Geometry check sheet. Reference: the model listing, model coordinates, mm. Round coordinates to 2 decimals unless told otherwise and drop trailing zeros. Write each loop counter-clockwise with the first axis right and the second up, starting at its lowest first coordinate (ties: lowest second). Pieces come first, ordered by that corner, then holes.
Item 1: Cross-section at B-B (z = 83.5). Enter the section's corners in (x, y), then the cut area to 3 significant figures.
Item 2: Depth check by flat-ended pin: P1, Ø18, axis at x = 0, y = 0, coming from the -Z side; P2, Ø1, axis at x = -10, z = 80.5, coming from the -Y side; P3, Ø12, axis at y = -12.5, z = 71, coming from the +X side; P4, Ø5, axis at x = 0, y = 0, coming from the +Z side. Enter the tip coordinate at first touch or a pass-through.
Item 3: Cross-section at A-A (x = 0). State how many separate pieces and enclosed holes the cut face has, then the cut area to 3 significant figures.
Item 4: Scan lines: probe 1 along X at (y, z) = (-0.5, 69); probe 2 along Y at (x, z) = (0, 149.75); probe 3 along Y at (x, z) = (0, 76.5). Record each from-to range of solid material in increasing order.
from build123d import *

# Parameters (mm, degrees)
F0_R      = 25.4
F1_DEPTH  = 152.5
F2_T      = -2.5
F3_R      = 6.5
F4_DEPTH  = 150
F5_T      = -2.5
F6_R      = 13.75
F7_DEPTH  = 12
F8_R      = 11.25
F11_DEPTH = 10
F12_R     = 25.4
F13_DEPTH = 2.5
F14_R     = 13.75
F15_DEPTH = 12.5
F16_R     = 11.25
F17_DEPTH = 10
F18_R     = 4
F19_DEPTH = 142.501
F20_R     = 3
F21_DEPTH = 25


# Not quite as in the source:
# - a fillet or chamfer that OpenCascade refuses, or shapes differently, is made with other operations: its cross-section is extruded or revolved along the edge and cut away or added


with BuildPart() as f1:
    # F0 (on Top) → F1 (new body)
    with BuildSketch(Plane.XY):
        Circle(F0_R)
    extrude(amount=F1_DEPTH)

    # F2
    f2_openings = [f1.faces().sort_by_distance(p)[0] for p in [
        (0, 0, 152.5),
    ]]
    offset(amount=F2_T, openings=f2_openings)

    # F3 (on face) → F4 (join)
    with BuildSketch(Plane.XY.offset(2.5)):
        Circle(F3_R)
    extrude(amount=F4_DEPTH)

    # F5: a shell. OpenCascade refuses it in one call, so the cavity is built on its own and cut out:
    # the body offset inwards by the wall thickness, plus a prism from it out through each open face.
    f5_core = offset(f1.part, amount=F5_T, kind=Kind.INTERSECTION, mode=Mode.PRIVATE)
    f5_exits = [f5_core.faces().sort_by_distance(p)[0] for p in [
        (0, 0, 150),
    ]]
    add(f5_core, mode=Mode.SUBTRACT)
    extrude(f5_exits, amount=-F5_T, mode=Mode.SUBTRACT)

    # F6 (on face) → F7 (join)
    with BuildSketch(Plane(origin=(0, 0, 0), x_dir=(1, 0, 0), z_dir=(0, 0, -1))):
        Circle(F6_R)
    extrude(amount=-F7_DEPTH)

    # F9: fillet of radius 10 on 1 edges, made by hand

    # F9_s1 → F9_t2 (revolve)
    with BuildSketch(Plane.XZ):
        with BuildLine():
            ThreePointArc((22.9, 12.4638095124), (20.2654599313, 5.6999348832), (13.75, 2.5))
            Line((13.75, 2.5), (22.9, 2.5))
            Line((22.9, 2.5), (22.9, 12.4638095124))
        make_face()
    revolve(axis=Axis((0, 0, 2.5), (0, 0, -1)))

    # F10: fillet of radius 8 on 1 edges, made by hand

    # F10_s1 → F10_t2 (revolve)
    with BuildSketch(Plane.XZ):
        with BuildLine():
            ThreePointArc((13.75, 12), (8.5839202169, 14.5796013539), (6.5, 19.964766161))
            Line((6.5, 19.964766161), (6.5, 12))
            Line((6.5, 12), (13.75, 12))
        make_face()
    revolve(axis=Axis((0, 0, 12), (0, 0, -1)))

    # F8 (on face) → F11 (cut)
    with BuildSketch(Plane(origin=(0, 0, 0), x_dir=(1, 0, 0), z_dir=(0, 0, -1))):
        Circle(F8_R)
    extrude(amount=-F11_DEPTH, mode=Mode.SUBTRACT)

    # F12 (on face) → F13 (join)
    with BuildSketch(Plane.XY.offset(152.5)):
        Circle(F12_R)
    extrude(amount=-F13_DEPTH)

    # F14 (on face) → F15 (join)
    with BuildSketch(Plane.XY.offset(152.5)):
        Circle(F14_R)
    extrude(amount=-F15_DEPTH)

    # F16 (on face) → F17 (cut)
    with BuildSketch(Plane.XY.offset(152.5)):
        Circle(F16_R)
    extrude(amount=-F17_DEPTH, mode=Mode.SUBTRACT)

    # F18 (on face) → F19 (cut, through all)
    with BuildSketch(Plane.XY.offset(142.5)):
        Circle(F18_R)
    extrude(amount=-F19_DEPTH, mode=Mode.SUBTRACT)

    # F20 (on face) → F21 (cut)
    with BuildSketch(Plane.XY.offset(152.5)):
        with Locations((18.1747831392, 0)):
            Circle(F20_R)
    extrude(amount=-F21_DEPTH, mode=Mode.SUBTRACT)


solid = f1.part
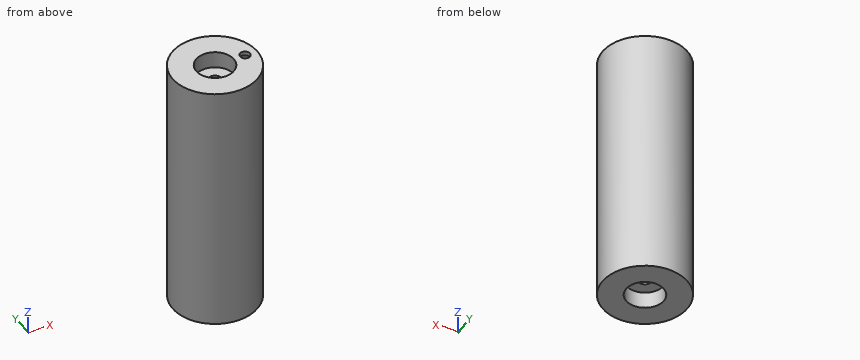
Resolved:
1. outline: circle Ø50.8 at (0, 0); circle Ø13 at (0, 0); hole circle Ø45.8 at (0, 0); hole circle Ø8 at (0, 0)
1. area: 462 mm2
2. P1: stops at z = 10
2. P2: stops at y = -23.56
2. P3: stops at x = 24.55
2. P4: passes through
3. separate pieces: 2
3. enclosed holes: 2
3. area: 1,750 mm2
4. probe 1: x = -25.4 to -22.89, -6.48 to -3.97, 3.97 to 6.48, 22.89 to 25.4
4. probe 2: y = -25.4 to -22.9, -13.75 to -11.25, 11.25 to 13.75, 22.9 to 25.4
4. probe 3: y = -25.4 to -22.9, -6.5 to -4, 4 to 6.5, 22.9 to 25.4
